from build123d import *

# Parameters (mm, degrees)
F1_DEPTH = 15
F3_DEPTH = 3.5
F4_SIZE  = 1
F5_R     = 2
F6_SIZE  = 0.5


with BuildPart() as f1:
    # F0 (on Top) → F1 (new body)
    with BuildSketch(Plane.XY):
        Polygon((-21, 1), (-20, 0), (-17.5, 0), (-17, 0), (-17, -7), (-17.5, -7.5), (-17.5, -10), (-18.5, -10), (-18.5, -10.5), (-16.761138632, -12.238861368), (-15.761138632, -12.238861368), (-13.8, -7), (-13.8, -2), (0, -2), (13.8, -2), (13.8, -7), (15.761138632, -12.238861368), (16.761138632, -12.238861368), (18.5, -10.5), (18.5, -10), (17.5, -10), (17.5, -7.5), (17, -7), (17, 0), (17.5, 0), (20, 0), (21, 1), (21, 3), (20, 4), (0, 4), (-20, 4), (-21, 3), align=None)
        Polygon((-17.5, -10), (-17.5, -7.5), (-18.5, -8.5), (-18.5, -10), align=None)
        Polygon((18.5, -8.5), (17.5, -7.5), (17.5, -10), (18.5, -10), align=None)
    extrude(amount=F1_DEPTH)

    # F2 (on face) → F3 (join)
    with BuildSketch(Plane.XY.offset(15)):
        Polygon((-20, 0), (-17, 0), (17, 0), (20, 0), (21, 1), (21, 3), (20, 4), (-20, 4), (-21, 3), (-21, 1), align=None)
    extrude(amount=F3_DEPTH)

    # F4
    f4_edges = [f1.edges().sort_by_distance(p)[0] for p in [
        (0, 0, 18.5),
        (20.5, 0.5, 18.5),
        (21, 2, 18.5),
        (20.5, 3.5, 18.5),
        (0, 4, 18.5),
        (-20.5, 3.5, 18.5),
        (-21, 2, 18.5),
        (-20.5, 0.5, 18.5),
    ]]
    chamfer(f4_edges, length=F4_SIZE)

    # F5
    f5_edges = [f1.edges().sort_by_distance(p)[0] for p in [
        (-17, -3.5, 0),
        (-17, -3.5, 15),
        (17, -3.5, 0),
        (17, -3.5, 15),
    ]]
    fillet(f5_edges, radius=F5_R)

    # F6
    f6_edges = [f1.edges().sort_by_distance(p)[0] for p in [
        (-16, 0, 0),
        (-18.5, 0, 0),
        (-15, -2.5, 0),
        (-20.5, 0.5, 0),
        (-16, -6, 0),
        (-21, 2, 0),
        (-17.75, -7.75, 0),
        (-20.5, 3.5, 0),
        (-18.5, -9.5, 0),
        (0, 4, 0),
        (-17.630569, -11.369431, 0),
        (20.5, 3.5, 0),
        (-16.261139, -12.238861, 0),
        (21, 2, 0),
        (-14.780569, -9.619431, 0),
        (20.5, 0.5, 0),
        (-13.8, -4.5, 0),
        (18.5, 0, 0),
        (0, -2, 0),
        (16, 0, 0),
        (13.8, -4.5, 0),
        (15, -2.5, 0),
        (14.780569, -9.619431, 0),
        (16, -6, 0),
        (16.261139, -12.238861, 0),
        (17.75, -7.75, 0),
        (17.630569, -11.369431, 0),
        (18.5, -9.5, 0),
    ]]
    chamfer(f6_edges, length=F6_SIZE)


solid = f1.part
Read the model definition and answer for the solid it produces. Units are mm, in the model's axes. A direction names the side the tool comes from. Coordinates: 2 decimals unless noted, no trailing zeros. Loops run counter-clockwise (first coordinate to the right, second up) from the corner with the lowest first, then second, coordinate; pieces in that order, holes last.
Q1. Consider probe 1 along X at (y, z) = (-6.5, 7.5); probe 2 along Y at (x, z) = (-11, 1); probe 3 along X at (y, z) = (-6.5, 13.75). Determine where each line is inside the solid, lowest interval first.
Q2. The part is cut by section D-D on z = 6.25. Write down the section's boundary in (x, y), and give its area (3 significant figures).
Q3. The part is cut by section C-C on x = 8.5. Write down the section's boundary in (y, z), and give its area (3 significant figures).
Q4. Each of these flat-tipped pins is pushed along its axis until it touches: pin 1 Ø5.5 at (y, z) = (-5, 7) entering from +X; pin 2 Ø1 at (y, z) = (-9, 8.5) entering from +X; pin 3 Ø8.5 at (x, z) = (-4, 8.5) entering from -Y. Where does it stop, or does it pass through?
Q5. The mould has two halves that part along Y. Classify faces 4 (the face through (17.08, -7.43, 0.25)), 5 (the face through (-15.03, -9.57, 0.25)), 6 (the face through (16.4, -3.2, 0.57)), 7 (the face through (0, 2, 18.5)): +Y half, -Y half, draft (parallel to the pull), parting line (faces both ways), or undercut.
Q6. The part is cut by section B-B on z = 17. Write down the section's boundary in (x, y), and give its area (3 significant figures).
Q7. Which of the six approach directions +Z, -Z, +X, -X, +Y, -Y give full straight-line access (tool end or side, diameter ignored) to faces 1 (the face through (0, -2, 8)), 2 (the face through (-18.5, -9, 8)), 3 (the face through (15, -9.49, 0.25))?
Q8. The part is cut by section A-A on y = -4. Write down the section's boundary in (x, z), and give its area (3 significant figures).
Results below:
1. probe 1: x = -17 to -13.8, 13.8 to 17
1. probe 2: y = -2 to 4
1. probe 3: x = -16.85 to -13.8, 13.8 to 16.85
2. outline: (-21, 1) - (-20, 0) - (-17, 0) - (-17, -7) - (-18.5, -8.5) - (-18.5, -10.5) - (-16.76, -12.24) - (-15.76, -12.24) - (-13.8, -7) - (-13.8, -2) - (13.8, -2) - (13.8, -7) - (15.76, -12.24) - (16.76, -12.24) - (18.5, -10.5) - (18.5, -8.5) - (17, -7) - (17, 0) - (20, 0) - (21, 1) - (21, 3) - (20, 4) - (-20, 4) - (-21, 3) - close
2. area: 300 mm2
3. outline: (-2, 0.5) - (-1.5, 0) - (3.5, 0) - (4, 0.5) - (4, 17.5) - (3, 18.5) - (1, 18.5) - (0, 17.5) - (0, 15) - (-2, 15) - close
3. area: 103 mm2
4. pin 1: stops at x = 17.75
4. pin 2: stops at x = 18.5
4. pin 3: stops at y = -2
5. face 4: undercut
5. face 5: -Y half
5. face 6: undercut
5. face 7: draft
6. outline: (-21, 1) - (-20, 0) - (20, 0) - (21, 1) - (21, 3) - (20, 4) - (-20, 4) - (-21, 3) - close
6. area: 166 mm2
7. face 1: +Z, -Z, -Y
7. face 2: +Z, -Z, -X, -Y
7. face 3: -Z, -Y
8. outline: (-17, 2) arc R2 ccw to (-15, 0) - (-14.3, 0) - (-13.8, 0.5) - (-13.8, 15) - (-15, 15) arc R2 ccw to (-17, 13) - close; (13.8, 0.5) - (14.3, 0) - (15, 0) arc R2 ccw to (17, 2) - (17, 13) arc R2 ccw to (15, 15) - (13.8, 15) - close
8. area: 92.3 mm2
